Part model, mm, in its own coordinate system. Face numbers are marked on the shaded views. A direction names the side the tool comes from. Round coordinates to 2 decimals unless told otherwise and drop trailing zeros. Write each loop counter-clockwise with the first axis right and the second up, starting at its lowest first coordinate (ties: lowest second). Pieces come first, ordered by that corner, then holes.
1) Saw through at D-D on x = 6. Write the cut outline in (y, z).
2) Flat gauge pins, fed straight in: pin 1 (10 mm diameter, centred on x = 11, z = -0.5, fed in from +Y); pin 2 (1.5 mm diameter, centred on y = -16.5, z = -7, fed in from +X); pin 3 (8 mm diameter, centred on x = 21.5, z = 2, fed in from -Y); pin 4 (2 mm diameter, centred on x = 20.75, z = -8.5, fed in from -Y). Where does each tip first touch, or does it go through?
3) Saw through at C-C on y = -17.8. Write the cut outline in (x, z), and give its area (3 significant figures).
4) Saw through at B-B on z = 0. Write the cut outline in (x, y).
5) Pull direction Z, two halves, no side cores. Call the marked faces 1, 2 and 3: +Z half, -Z half, draft (parallel to the pull), parting line (faces both ways), or undercut.
6) Which spindle directions (+Z, -Z, +X, -X, +Y, -Y) get a long thin tool onto all of the face, cutting with end or side? Do the marked faces 4 and 5. Say none if no direction does.
7) Drill centre lines: L1, parallel to Y at x = 2.2, z = 0; L2, parallel to Y at x = 1.7, z = -8; L3, parallel to Y at x = 27, z = -10.75. Where is each one in solid material? Low to high.
8) Saw through at A-A on y = -10.85. Write the cut outline in (x, z), and give its area (3 significant figures).
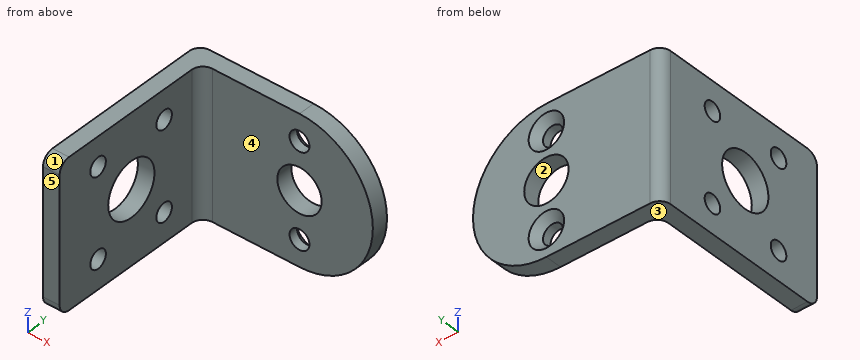
```python
from build123d import *

# Parameters (mm, degrees)
EXTRUDE_1_DEPTH           = 13.25
CUT_EXTRUDE_2_DEPTH       = 40
SKETCH_5_R                = 1.65
SKETCH_5_R_2              = 4.9
CUT_EXTRUDE_4_DEPTH       = 40
FILLET_1_R                = 2
SKETCH_7_R                = 4
CUT_EXTRUDE_5_DEPTH       = 10
HOLE_WIZARD_1_D           = 3.6
HOLE_WIZARD_1_DEPTH       = 8
HOLE_WIZARD_1_CSINK_D     = 6.4
HOLE_WIZARD_1_CSINK_ANGLE = 90
HOLE_WIZARD_1_TIP         = 1.081549114
HOLE_WIZARD_2_D           = 3.6
HOLE_WIZARD_2_DEPTH       = 8
HOLE_WIZARD_2_CSINK_D     = 6.4
HOLE_WIZARD_2_CSINK_ANGLE = 90
HOLE_WIZARD_2_TIP         = 1.081549114


with BuildPart() as part:
    # 草图1 → 凸台-拉伸1 (new, symmetric)
    with BuildSketch(Plane.XY):
        with BuildLine():
            Line((0, -33), (0, -2))
            ThreePointArc((0, -2), (0.585786438, -0.585786438), (2, 0))
            Line((2, 0), (50, 0))
            Line((50, 0), (50, -3))
            Line((50, -3), (5, -3))
            ThreePointArc((5, -3), (3.585786438, -3.585786438), (3, -5))
            Line((3, -5), (3, -33))
            Line((3, -33), (0, -33))
        make_face()
    extrude(amount=EXTRUDE_1_DEPTH, both=True)

    # 草图3 → 切除-拉伸2 (cut)
    with BuildSketch(Plane.XZ.offset(3)):
        with BuildLine():
            Line((20.75, 13.25), (50, 13.25))
            Line((50, 13.25), (50, -13.25))
            Line((50, -13.25), (20.75, -13.25))
            ThreePointArc((20.75, -13.25), (34, 0), (20.75, 13.25))
        make_face()
    extrude(amount=-CUT_EXTRUDE_2_DEPTH, mode=Mode.SUBTRACT)

    # 草图5 → 切除-拉伸4 (cut)
    with BuildSketch(Plane.ZY):
        with Locations((8, -10.85)):
            Circle(SKETCH_5_R)
        with Locations((8, -24.85)):
            Circle(SKETCH_5_R)
        with Locations((-8, -24.85)):
            Circle(SKETCH_5_R)
        with Locations((-8, -10.85)):
            Circle(SKETCH_5_R)
        with Locations((0, -17.8)):
            Circle(SKETCH_5_R_2)
    extrude(amount=-CUT_EXTRUDE_4_DEPTH, mode=Mode.SUBTRACT)

    # 圆角1
    fillet_1_edges = [part.edges().sort_by_distance(p)[0] for p in [
        (1.5, -33, 13.25),
        (1.5, -33, -13.25),
    ]]
    fillet(fillet_1_edges, radius=FILLET_1_R)

    # 草图7 → 切除-拉伸5 (cut)
    with BuildSketch(Plane(origin=(0, 0, 0), x_dir=(1, 0, 0), z_dir=(0, 1, 0))):
        with Locations(Location((20.75, 0, 0), (0, 0, 270))):
            Circle(SKETCH_7_R)
    extrude(amount=-CUT_EXTRUDE_5_DEPTH, mode=Mode.SUBTRACT)

    # 打孔尺寸开槽半沉头螺钉的类型1
    with Locations(Plane(origin=(0, 0, 0), x_dir=(1, 0, 0), z_dir=(0, 1, 0))):
        with Locations((20.75, -8.5)):
            CounterSinkHole(HOLE_WIZARD_1_D / 2, HOLE_WIZARD_1_CSINK_D / 2, depth=HOLE_WIZARD_1_DEPTH, counter_sink_angle=HOLE_WIZARD_1_CSINK_ANGLE)
            with Locations((0, 0, -(HOLE_WIZARD_1_DEPTH + HOLE_WIZARD_1_TIP / 2))):  # 118° drill point
                Cone(0, HOLE_WIZARD_1_D / 2, HOLE_WIZARD_1_TIP, mode=Mode.SUBTRACT)

    # 打孔尺寸开槽半沉头螺钉的类型2
    with Locations(Plane(origin=(0, 0, 0), x_dir=(1, 0, 0), z_dir=(0, 1, 0))):
        with Locations((20.75, 8.5)):
            CounterSinkHole(HOLE_WIZARD_2_D / 2, HOLE_WIZARD_2_CSINK_D / 2, depth=HOLE_WIZARD_2_DEPTH, counter_sink_angle=HOLE_WIZARD_2_CSINK_ANGLE)
            with Locations((0, 0, -(HOLE_WIZARD_2_DEPTH + HOLE_WIZARD_2_TIP / 2))):  # 118° drill point
                Cone(0, HOLE_WIZARD_2_D / 2, HOLE_WIZARD_2_TIP, mode=Mode.SUBTRACT)


solid = part.part
```
Completed:
1. outline: (-3, -13.25) - (0, -13.25) - (0, 13.25) - (-3, 13.25) - close
2. pin 1: stops at y = 0
2. pin 2: stops at x = 3
2. pin 3: stops at y = -3
2. pin 4: passes through
3. outline: (0, -13.25) - (3, -13.25) - (3, -4.9) - (0, -4.9) - close; (0, 4.9) - (3, 4.9) - (3, 13.25) - (0, 13.25) - close
3. area: 50.1 mm2
4. outline: (0, -33) - (3, -33) - (3, -22.7) - (0, -22.7) - close; (0, -12.9) - (3, -12.9) - (3, -5) arc R2 cw to (5, -3) - (16.75, -3) - (16.75, 0) - (2, 0) arc R2 ccw to (0, -2) - close; (24.75, -3) - (34, -3) - (34, 0) - (24.75, 0) - close
5. face 1: +Z half
5. face 2: undercut
5. face 3: -Z half
6. face 4: +Z, -Z, +X, -Y
6. face 5: +Z, -Z, +X, -X, -Y
7. L1: y = -33 to -22.7, -12.9 to 0
7. L2: y = -33 to -26.5, -23.2 to -12.5, -9.2 to -0.02
7. L3: y = -3 to 0
8. outline: (0, -13.25) - (3, -13.25) - (3, -9.65) - (0, -9.65) - close; (0, -6.35) - (3, -6.35) - (3, 6.35) - (0, 6.35) - close; (0, 9.65) - (3, 9.65) - (3, 13.25) - (0, 13.25) - close
8. area: 59.7 mm2
